Source: three-view drawing plus pictorial views. Frame: mm from the lowest corner of the part. Coordinates: 2 decimals unless noted, no trailing zeros. Loops run counter-clockwise (first coordinate to the right, second up) from the corner with the lowest first, then second, coordinate; pieces in that order, holes last.
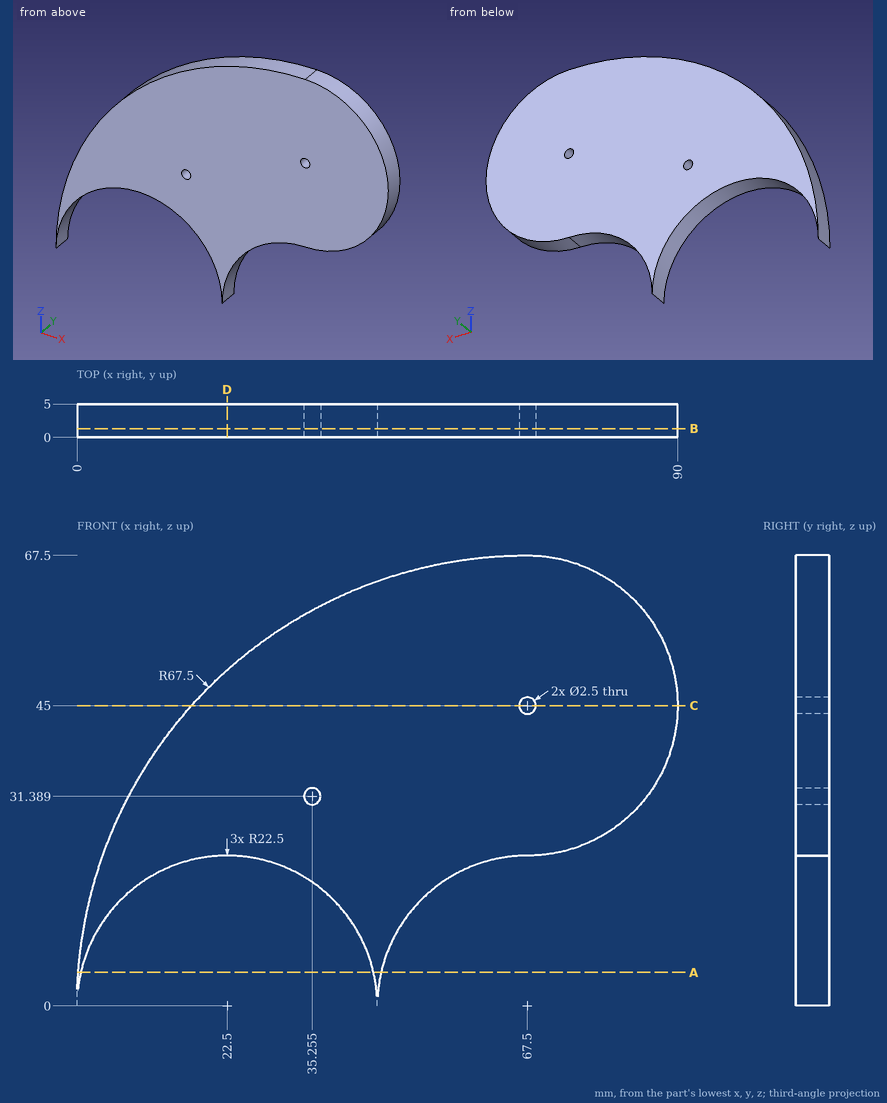
Q1. Section B-B, the plane y = 1.3. Return the cut outline in (x, z) (3 decimals), plus the area to 3 significant figures.
Q2. Section C-C, the plane z = 45. Return the cut outline in (x, y).
Q3. Section A-A, the plane z = 5. Return the cut outline in (x, y).
Q4. Section D-D, the plane x = 22.5. Return the cut outline in (y, z).
Q5. Line query: line 1 along Z through (x, y) = (67.5, 1.6); line 2 along X through (y, z) = (1.6, 44); line 3 along Z through (x, y) = (66.5, 2.1). Output: solid intervals per line, ascending.
Q6. Contact query for flat-ended pins moving along their axis: pin 1 Ø1.5 at (x, z) = (67.5, 45) entering from +Y; pin 2 Ø1 at (y, z) = (3, 16) entering from -X; pin 3 Ø3 at (x, y) = (78.5, 1.5) entering from -Z; pin 4 Ø1.5 at (y, z) = (3.5, 27) entering from +X. Output: stop coordinate, or through.
Derived:
1. outline: (0, 0) arc R22.5 cw to (45, 0) arc R22.5 cw to (67.5, 22.5) arc R22.5 ccw to (67.5, 67.5) arc R67.5 ccw to start; hole circle Ø2.5 at (35.255, 31.389); hole circle Ø2.5 at (67.5, 45)
1. area: 3,170 mm2
2. outline: (17.19, 0) - (66.25, 0) - (66.25, 5) - (17.19, 5) - close; (68.75, 0) - (90, 0) - (90, 5) - (68.75, 5) - close
3. outline: (0.19, 0) - (0.56, 0) - (0.56, 5) - (0.19, 5) - close; (44.44, 0) - (45.56, 0) - (45.56, 5) - (44.44, 5) - close
4. outline: (0, 22.5) - (5, 22.5) - (5, 50.31) - (0, 50.31) - close
5. line 1: z = 22.5 to 43.75, 46.25 to 67.5
5. line 2: x = 16.31 to 66.75, 68.25 to 89.98
5. line 3: z = 22.48 to 44.25, 45.75 to 67.49
6. pin 1: passes through
6. pin 2: stops at x = 1.8
6. pin 3: stops at z = 24.6
6. pin 4: stops at x = 81.95
